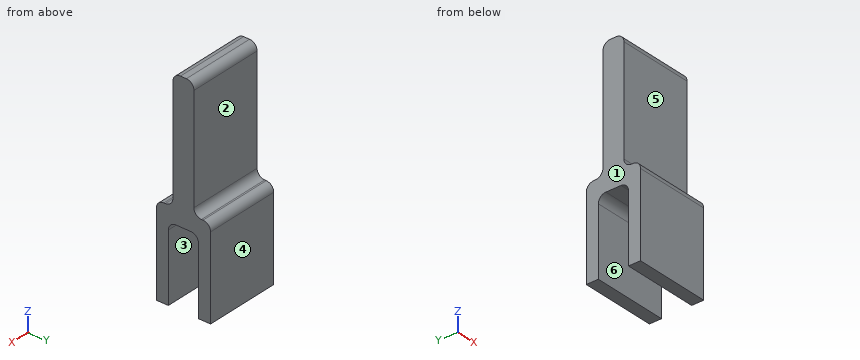
from build123d import *

# Parameters (mm, degrees)
SKETCH_1_W          = 6.6
SKETCH_1_H          = 3.6
SKETCH_1_W_2        = 5
SKETCH_1_H_2        = 2
EXTRUDE_1_DEPTH     = 5
CUT_EXTRUDE_2_REACH = 8.255
SKETCH_2_W          = 0.8
SKETCH_2_H          = 3.6
SKETCH_3_W          = 5
SKETCH_3_H          = 3.6
EXTRUDE_1_2_DEPTH   = 1
SKETCH_4_W          = 5
SKETCH_4_H          = 1.393036208
EXTRUDE_2_DEPTH     = 8
FILLET_1_R          = 0.5


with BuildPart() as part:
    # Sketch 1 → Extrude 1 (new body)
    with BuildSketch(Plane.XY):
        Rectangle(SKETCH_1_W, SKETCH_1_H)
        Rectangle(SKETCH_1_W_2, SKETCH_1_H_2, mode=Mode.SUBTRACT)
    extrude(amount=EXTRUDE_1_DEPTH)

    # Sketch 2 → Cut-Extrude 2 (cut, up to next)
    with BuildSketch(Plane.XY.offset(5), mode=Mode.PRIVATE) as cut_extrude_2_sk1:
        with Locations((-2.9, 0)):
            Rectangle(SKETCH_2_W, SKETCH_2_H)
    cut_extrude_2_tool1 = extrude(cut_extrude_2_sk1.sketch, amount=-CUT_EXTRUDE_2_REACH, mode=Mode.PRIVATE) & part.part
    # Sketch 2 → Cut-Extrude 2 (cut, up to next)
    with BuildSketch(Plane.XY.offset(5), mode=Mode.PRIVATE) as cut_extrude_2_sk2:
        with Locations((2.9, 0)):
            Rectangle(SKETCH_2_W, SKETCH_2_H)
    cut_extrude_2_tool2 = extrude(cut_extrude_2_sk2.sketch, amount=-CUT_EXTRUDE_2_REACH, mode=Mode.PRIVATE) & part.part
    add(cut_extrude_2_tool1.solids().sort_by_distance((-2.9, 0, 5))[0], mode=Mode.SUBTRACT)
    add(cut_extrude_2_tool2.solids().sort_by_distance((2.9, 0, 5))[0], mode=Mode.SUBTRACT)


with BuildPart() as cut_extrude_2_piece_1:
    # of the separate pieces the step leaves, piece 1, a body of its own (cut_extrude_2_pieces)
    add(part.part.solids().sort_by_distance((2.5, -1.8, 0))[0])



with BuildPart() as cut_extrude_2_piece_2:
    # of the separate pieces the step leaves, piece 2, a body of its own (cut_extrude_2_pieces)
    add(part.part.solids().sort_by_distance((-2.5, 1.8, 0))[0])


with BuildPart() as cut_extrude_2_piece_1_1:
    add(cut_extrude_2_piece_1.part)

    add(cut_extrude_2_piece_2.part)  # Extrude 1 2 merges Cut-Extrude 2 piece 2
    # Sketch 3 → Extrude 1 2 (add)
    with BuildSketch(Plane.XY.offset(5)):
        Rectangle(SKETCH_3_W, SKETCH_3_H)
    extrude(amount=EXTRUDE_1_2_DEPTH)

    # Sketch 4 → Extrude 2 (add)
    with BuildSketch(Plane.XY.offset(6)):
        Rectangle(SKETCH_4_W, SKETCH_4_H)
    extrude(amount=EXTRUDE_2_DEPTH)

    # Fillet 1
    fillet_1_edges = [cut_extrude_2_piece_1_1.edges().sort_by_distance(p)[0] for p in [
        (0, -1.8, 6),
        (0, 1.8, 6),
        (0, 1, 5),
        (0, -1, 5),
        (0, 0.696518104, 6),
        (0, -0.696518104, 6),
        (0, 0.696518104, 14),
        (0, -0.696518104, 14),
    ]]
    fillet(fillet_1_edges, radius=FILLET_1_R)


solid = cut_extrude_2_piece_1_1.part
Model file for the job. Use its own axes, mm. Face numbers are marked on the shaded views. A direction names the side the tool comes from. Give positions to 0.01 mm unless a question says otherwise; leave off trailing zeros. Order: outer loops, then holes, each group sorted by start corner. A loop starts at its lowest first (then second) coordinate and runs counter-clockwise, first axis right, second up. Notation, with made-up numbers: M 19,48 L 26,48 A32 ccw 26,86 Z; hole C -6.75,-29.75 d10. An arc over 180 degrees is marked long. Put each result on its own line as item: value. Start each with the question number.
(1) Drill centre lines: L1, parallel to Y at x = 1.35, z = 1; L2, parallel to Y at x = -0.4, z = 11; L3, parallel to Z at x = 1.9, y = 1.35. Where is each one in solid material? Low to high. Write a range as [from, to].
(2) Tool access for the marked faces 1, 2 and 3: list every direction of +Z, -Z, +X, -X, +Y, -Y with a clear straight run to the whole face (end or side of a thin tool).
(3) Band-saw the part on D-D on y = -0.05. Give the cut face in (x, z), then the cut area to 3 significant figures.
(4) Band-saw the part on C-C on z = 4.75. Give the cut face in (x, y).
(5) Pull direction Y, two halves, no side cores. Call the marked faces 4, 5 and 6: released by +Y, released by -Y, zero draft, split by the parting line, or undercut.
(6) Pin check, flat tips, straight feed: pin 1 Ø0.8 at (x, y) = (0.5, 0) entering from -Z; pin 2 Ø2 at (y, z) = (-0.5, 3.5) entering from +X; pin 3 Ø3 at (x, z) = (2, 12) entering from -Y. Stop position of each tip, or through.
(7) Band-saw the part on A-A on z = 1.75. Give the cut face in (x, y).
(8) Band-saw the part on B-B on x = 0.3. Give the cut face in (y, z), then the cut area to 3 significant figures.
Results below:
1. L1: y = [-1.8, -1], [1, 1.8]
1. L2: y = [-0.7, 0.7]
1. L3: z = [0, 6]
2. face 1: +Z, -Z, -X, +Y, -Y
2. face 2: +Z, +X, -X, +Y
2. face 3: -Z, +X, -X
3. outline: M -2.5,5 L 2.5,5 L 2.5,14 L -2.5,14 Z
3. area: 45.0 mm2
4. outline: M -2.5,-1.8 L 2.5,-1.8 L 2.5,-0.93 L -2.5,-0.93 Z; M -2.5,0.93 L 2.5,0.93 L 2.5,1.8 L -2.5,1.8 Z
5. face 4: released by +Y
5. face 5: released by -Y
5. face 6: undercut
6. pin 1: stops at z = 5
6. pin 2: stops at x = 2.5
6. pin 3: stops at y = -0.7
7. outline: M -2.5,-1.8 L 2.5,-1.8 L 2.5,-1 L -2.5,-1 Z; M -2.5,1 L 2.5,1 L 2.5,1.8 L -2.5,1.8 Z
8. outline: M -1.8,0 L -1,0 L -1,4.5 A0.5 cw -0.5,5 L 0.5,5 A0.5 cw 1,4.5 L 1,0 L 1.8,0 L 1.8,5.5 A0.5 ccw 1.3,6 L 1.2,6 A0.5 cw 0.7,6.5 L 0.7,13.5 A0.5 ccw 0.2,14 L -0.2,14 A0.5 ccw -0.7,13.5 L -0.7,6.5 A0.5 cw -1.2,6 L -1.3,6 A0.5 ccw -1.8,5.5 Z
8. area: 22.7 mm2
